```python
from build123d import *

# Parameters (mm, degrees)
SKETCH2_W           = 94.751202958
SKETCH2_H           = 91.163886598
BOSS_EXTRUDE1_DEPTH = 45
CUT_EXTRUDE3_DEPTH  = 35
FILLET2_SIZE        = 7.5
FILLET3_R           = 7.5


with BuildPart() as part:
    # Sketch2 → Boss-Extrude1 (new body)
    with BuildSketch(Plane.XY):
        with Locations((-304.121373084, 372.346881372)):
            Rectangle(SKETCH2_W, SKETCH2_H)
    extrude(amount=BOSS_EXTRUDE1_DEPTH)

    # Sketch5 → Cut-Extrude3 (cut)
    with BuildSketch(Plane.XY.offset(45)):
        with BuildLine():
            Line((-371.329773575, 356.337977129), (-320.45664172, 351.735015891))
            ThreePointArc((-320.45664172, 351.735015891), (-313.755539426, 347.87500284), (-306.221453805, 346.130862205))
            Line((-306.221453805, 346.130862205), (-238.931197352, 340.740456843))
            Line((-238.931197352, 340.740456843), (-238.931197352, 403.953305901))
            Line((-238.931197352, 403.953305901), (-306.221453805, 398.562900539))
            ThreePointArc((-306.221453805, 398.562900539), (-313.755539426, 396.818759904), (-320.45664172, 392.958746853))
            Line((-320.45664172, 392.958746853), (-371.329773575, 388.355785615))
            Line((-371.329773575, 388.355785615), (-371.329773575, 356.337977129))
        make_face()
    extrude(amount=-CUT_EXTRUDE3_DEPTH, mode=Mode.SUBTRACT)

    # Fillet2
    # a fillet whose section is not a circle: 7.5 mm, written as the material it takes off along each edge
    with BuildSketch(Plane(origin=(-351.496974563, 326.764938073, -18.75), x_dir=(0, 1, 0), z_dir=(0, 0, 1)), Plane(origin=(-351.496974563, 417.928824671, -18.75), x_dir=(1, 0, 0), z_dir=(0, 0, 1))) as fillet2_piece_1:
        with BuildLine():
            add(Edge.make_bspline([(FILLET2_SIZE, 0), (6.238514613, 0), (4.977029227, 0), (2.196699141, -0.537689399), (0.537689399, -2.196699141), (0, -4.977029227), (0, -6.238514613), (0, -FILLET2_SIZE)], knots=[0, 0, 0, 0, 0, 0, 0.5, 0.5, 1, 1, 1, 1, 1, 1], degree=5))
            Line((0, -FILLET2_SIZE), (0, 0))
            Line((0, 0), (FILLET2_SIZE, 0))
        make_face()
    extrude(amount=82.5, mode=Mode.SUBTRACT)
    with BuildSketch(Plane(origin=(-351.496974563, 354.543520964, 10), x_dir=(0, -1, 0), z_dir=(0, 0, 1)), Plane(origin=(-351.496974563, 390.15024178, 65.523077256), x_dir=(0, 1, 0), z_dir=(0, 0, -1))) as fillet2_piece_2:
        with BuildLine():
            add(Edge.make_bspline([(8.209230902, 0), (6.849526251, 0), (5.4898216, 0), (2.507242029, 0.618786495), (0.842199494, 2.441282313), (0.494693995, 5.467487453), (0.617218509, 6.821660441), (0.739743023, 8.17583343)], knots=[0, 0, 0, 0, 0, 0, 0.5, 0.5, 1, 1, 1, 1, 1, 1], degree=5))
            Line((0.739743023, 8.17583343), (0, 0))
            Line((0, 0), (8.209230902, 0))
        make_face()
    extrude(amount=55.523077256, mode=Mode.SUBTRACT)
    with BuildSketch(Plane(origin=(-256.745771605, 417.928824671, -18.75), x_dir=(-1, 0, 0), z_dir=(0, 0, 1)), Plane(origin=(-256.745771605, 326.764938073, -18.75), x_dir=(0, 1, 0), z_dir=(0, 0, 1))) as fillet2_piece_3:
        with BuildLine():
            add(Edge.make_bspline([(FILLET2_SIZE, 0), (6.238514613, 0), (4.977029227, 0), (2.196699141, 0.537689399), (0.537689399, 2.196699141), (0, 4.977029227), (0, 6.238514613), (0, FILLET2_SIZE)], knots=[0, 0, 0, 0, 0, 0, 0.5, 0.5, 1, 1, 1, 1, 1, 1], degree=5))
            Line((0, FILLET2_SIZE), (0, 0))
            Line((0, 0), (FILLET2_SIZE, 0))
        make_face()
    extrude(amount=82.5, mode=Mode.SUBTRACT)
    with BuildSketch(Plane(origin=(-256.745771605, 342.167524916, 62.308062051), x_dir=(0, -1, 0), z_dir=(0, 0, -1)), Plane(origin=(-256.745771605, 402.526237828, 10), x_dir=(0, 1, 0), z_dir=(0, 0, 1))) as fillet2_piece_4:
        with BuildLine():
            add(Edge.make_bspline([(6.923224821, 0), (5.744187381, 0), (4.565149942, 0), (1.957575936, 0.472170808), (0.314348726, 1.989028329), (-0.364531688, 4.550572562), (-0.45867898, 5.725845114), (-0.552826273, 6.901117665)], knots=[0, 0, 0, 0, 0, 0, 0.5, 0.5, 1, 1, 1, 1, 1, 1], degree=5))
            Line((-0.552826273, 6.901117665), (0, 0))
            Line((0, 0), (6.923224821, 0))
        make_face()
    extrude(amount=52.308062051, mode=Mode.SUBTRACT)

    # Fillet3
    fillet3_edges = [part.edges().sort_by_distance(p)[0] for p in [
        (-320.45664172, 351.735015891, 27.5),
        (-320.45664172, 392.958746853, 27.5),
    ]]
    fillet(fillet3_edges, radius=FILLET3_R)


solid = part.part
```
The listing builds one solid part. Answer for the finished solid, in the listing's coordinates (mm). A direction names the side the tool comes from. Give positions to 0.01 mm unless a question says otherwise; leave off trailing zeros. Order: outer loops, then holes, each group sorted by start corner. A loop starts at its lowest first (then second) coordinate and runs counter-clockwise, first axis right, second up.
1) Find section A-A on x = -276. Write down the section's boundary in (y, z).
Reported:
outline: (326.76, 0) - (417.93, 0) - (417.93, 45) - (400.98, 45) - (400.98, 10) - (343.71, 10) - (343.71, 45) - (326.76, 45) - close
2) For faces 1 (the face through (-256.746, 372, 4)), 2 (the face through (-320.648, 351.502, 27.255)), determine the directions among +Z, -Z, +X, -X, +Y, -Y from which every point of the face is accessible in a straight line to the end or side of a thin tool.
Reported:
face 1: +Z, -Z, +X, +Y, -Y
face 2: +Z, +X
3) Consider line 1 along Z through (x, y) = (-333.5, 383); line 2 along Y through (x, z) = (-304.5, 33.5); line 3 along Y through (x, z) = (-314, 13). Determine where each line is inside the solid, lowest interval first.
Reported:
line 1: z = 0 to 10
line 2: y = 326.76 to 345.99, 398.7 to 417.93
line 3: y = 326.76 to 347.97, 396.72 to 417.93
4) Find section B-B on y = 362. Write down the section's boundary in (x, z), then the cut area to 3 significant figures.
Reported:
outline: (-351.5, 0) - (-256.75, 0) - (-256.75, 10) - (-351.5, 10) - close
area: 948 mm2
5) Find section C-C on x = -294. Write down the section's boundary in (y, z).
Reported:
outline: (326.76, 0) - (417.93, 0) - (417.93, 45) - (399.54, 45) - (399.54, 10) - (345.15, 10) - (345.15, 45) - (326.76, 45) - close
6) Given P1, Ø1.5, axis at x = -321, y = 380, coming from the -Z side; P2, Ø1, axis at y = 394, z = 14.5, coming from the +X side, each flat-ended and moving along its own axis, determine where each tip first touches the part or whether it passes through.
Reported:
P1: stops at z = 0
P2: stops at x = -318.3
